Part print with two shaded views. Sizes in mm from the minimum x, y, z corner. A direction names the side the tool comes from. Round coordinates to 2 decimals unless told otherwise and drop trailing zeros. Order: outer loops, then holes, each group sorted by start corner. A loop starts at its lowest first (then second) coordinate and runs counter-clockwise, first axis right, second up. Notation, with made-up numbers: (67.25, 36.5) - (84.25, 36.5) arc R27 cw to (84.25, 65.5) - close; hole circle Ø3 at (46, 20). An arc over 180 degrees is marked (long way). Answer as CSV lines item,"result". Start each with the question number.
1. Band-saw the part on A-A on z = 1.75. List the corners of the cut face in (x, y).
2. Band-saw the part on D-D on y = 19.75. List the corners of the cut face in (x, z).
3. Band-saw the part on B-B on x = 17. List the corners of the cut face in (y, z).
4. Wall check: line 1 along Y through (x, z) = (16.25, 9.25); line 2 along Y through (x, z) = (4.5, 6.5); line 3 along X through (y, z) = (9, 3). Give the ranges that are in metal, low to high. Write a range as [from, to].
5. Pin check, flat tips, straight feed: pin 1 Ø1.2 at (x, y) = (9, 1) entering from -Z; pin 2 Ø1.2 at (y, z) = (1, 7) entering from +X; pin 3 Ø2 at (x, z) = (18.5, 1.5) entering from -Y. Stop position of each tip, or through.
6. 3-axis set-ups, long thin cutter, end or side, ignore diameter. For the marked faces 4, 5, 6, 7 and 8: which of +Z, -Z, +X, -X, +Y, -Y reach the whole face in a straight line?
7. Band-saw the part on C-C on x = 12.5. List the corners of the cut face in (y, z), then the cut area to 3 significant figures.
8. Pull direction Y, two halves, no side cores. Call the marked faces 1, 2 and 3: released by +Y, released by -Y, zero draft, split by the parting line, or undercut.
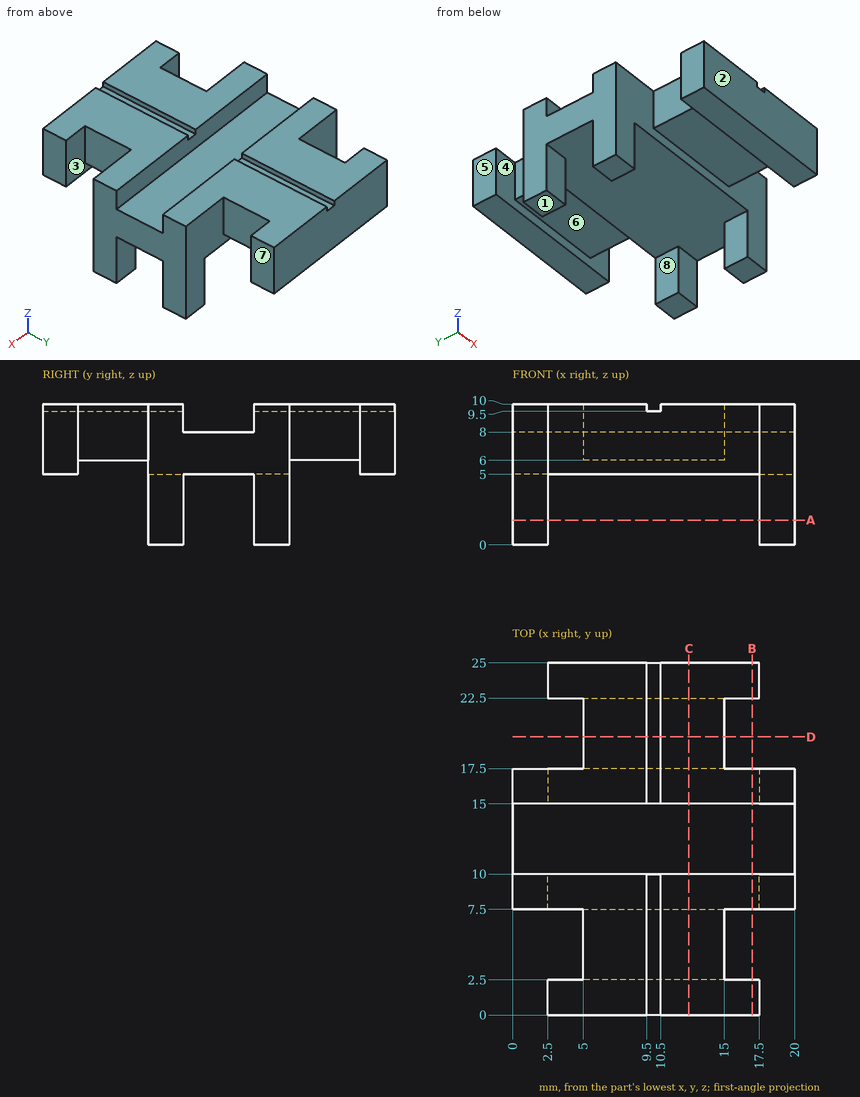
Reply:
1,outline,"(0, 7.5) - (2.5, 7.5) - (2.5, 10) - (0, 10) - close; (0, 15) - (2.5, 15) - (2.5, 17.5) - (0, 17.5) - close; (17.5, 7.5) - (20, 7.5) - (20, 10) - (17.5, 10) - close; (17.5, 15) - (20, 15) - (20, 17.5) - (17.5, 17.5) - close"
2,outline,"(5, 6) - (15, 6) - (15, 10) - (10.5, 10) - (10.5, 9.5) - (9.5, 9.5) - (9.5, 10) - (5, 10) - close"
3,outline,"(0, 5) - (2.5, 5) - (2.5, 10) - (0, 10) - close; (7.5, 5) - (17.5, 5) - (17.5, 10) - (15, 10) - (15, 8) - (10, 8) - (10, 10) - (7.5, 10) - close; (22.5, 5) - (25, 5) - (25, 10) - (22.5, 10) - close"
4,line 1,"y = [0, 2.5], [7.5, 10], [15, 17.5], [22.5, 25]"
4,line 2,"y = [0, 2.5], [7.5, 17.5], [22.5, 25]"
4,line 3,"x = [0, 2.5], [17.5, 20]"
5,pin 1,"stops at z = 5"
5,pin 2,"stops at x = 17.5"
5,pin 3,"stops at y = 7.5"
6,face 4,"-Z"
6,face 5,"+Z, -Z, -X, +Y"
6,face 6,"-Z, +X, -X"
6,face 7,"+Z, -Z, +X, +Y"
6,face 8,"-Z, +Y, -Y"
7,outline,"(0, 5) - (2.5, 5) - (2.5, 6) - (7.5, 6) - (7.5, 5) - (17.5, 5) - (17.5, 6) - (22.5, 6) - (22.5, 5) - (25, 5) - (25, 10) - (15, 10) - (15, 8) - (10, 8) - (10, 10) - (0, 10) - close"
7,area,"105 mm2"
8,face 1,"zero draft"
8,face 2,"released by -Y"
8,face 3,"undercut"
